Can you work these out from the drawing? Everything is in mm from the part's minimum corner. A direction names the side the tool comes from. Coordinates: 2 decimals unless noted, no trailing zeros. Write each loop counter-clockwise with the first axis right and the second up, starting at its lowest first coordinate (ties: lowest second). Pieces come first, ordered by that corner, then holes. Notation, with made-up numbers: (5.25, -0.75) -> (51.25, -0.75) arc R26 cw to (51.25, 35.25) -> close; hole circle Ø3 at (81, 16.25). An arc over 180 degrees is marked (long way). Use a Markdown table: item, result. Add a question column.
Item 1: Imagine slicing it at C-C, the plane y = 9. Write out the boundary of the cut face in (x, z), and give its area (4 significant figures).
Item 2: Imagine slicing it at A-A, the plane z = 5. Write out the boundary of the cut face in (x, y), and give its area (3 significant figures).
Item 3: If we mould it in two halves opening along X, with no side actions, what happens to the marked faces 1, 2, 3 and 4? For each: pulls with the +X half, pulls with the -X half, needs draft (parallel to the pull), parting line crosses it, or undercut.
Item 4: If I drill on line 1 along X through (y, z) = (5.5, 5.5); line 2 along Z through (x, y) = (5, 3.6); line 3 along Y through (x, z) = (3.75, 2.25), over which ranges is the centre line in solid material (lowest first)? Write a range as from..to.
Item 5: Imagine slicing it at B-B, the plane x = 5. Write out the boundary of the cut face in (y, z), and give its area (3 significant figures).
Item 6: Will these pins go through, and if not, where does the flat tip stop? pin 1 Ø5.5 at (x, z) = (5, 6) entering from +Y; pin 2 Ø6 at (y, z) = (1.5, 8.5) entering from -X; pin 3 Ø1 at (x, y) = (7.5, 2.5) entering from +Z.
Item 7: On a 3-axis mill with a long thin cutter (end or side, diameter ignored), from which of +Z, -Z, +X, -X, +Y, -Y can I reach the whole of each face in a straight line? I mean the marked faces 5, 6 and 7. Say none if no direction works.
Item 8: Imagine slicing it at D-D, the plane y = 1. Write out the boundary of the cut face in (x, z), and give its area (3 significant figures).
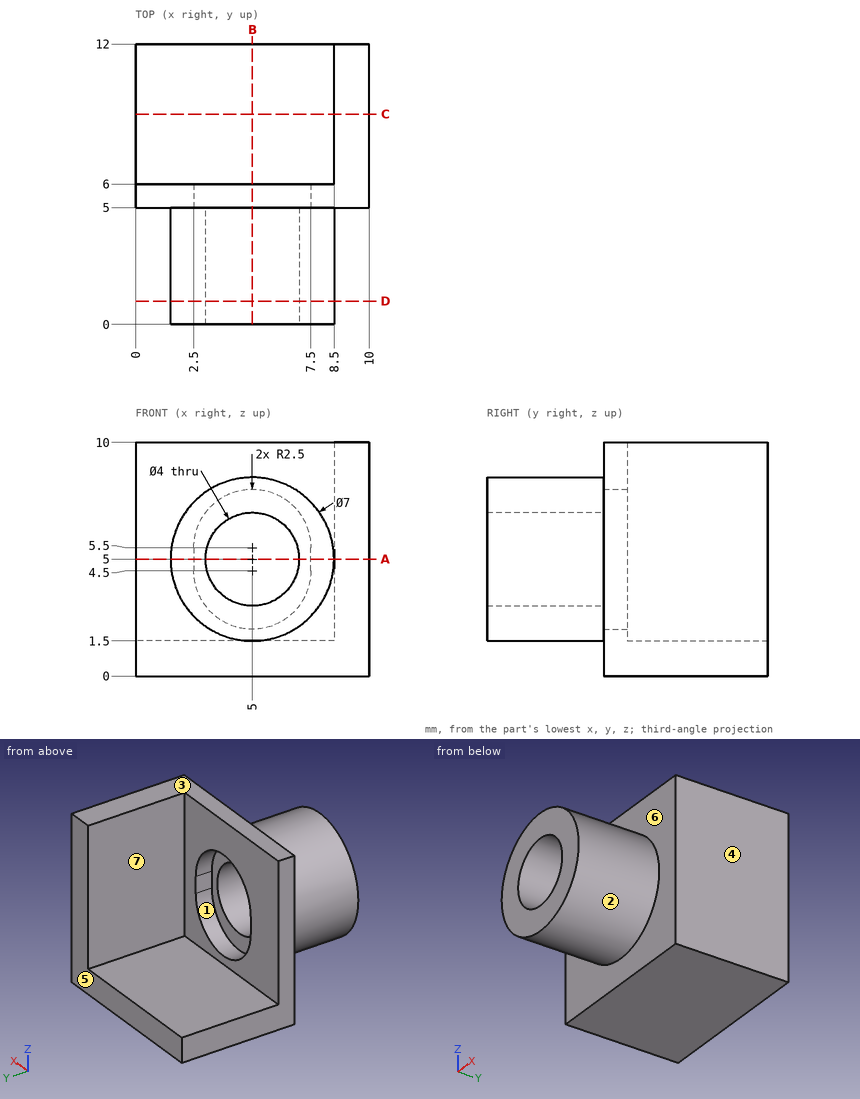
Ans:
| question | item | result |
|---|---|---|
| 1 | outline | (0, 0) -> (10, 0) -> (10, 10) -> (8.5, 10) -> (8.5, 1.5) -> (0, 1.5) -> close |
| 1 | area | 27.75 mm^2 |
| 2 | outline | (0, 5) -> (1.5, 5) -> (1.5, 0) -> (3, 0) -> (3, 5) -> (2.5, 5) -> (2.5, 6) -> (0, 6) -> close; (7, 0) -> (8.5, 0) -> (8.5, 5) -> (10, 5) -> (10, 12) -> (8.5, 12) -> (8.5, 6) -> (7.5, 6) -> (7.5, 5) -> (7, 5) -> close |
| 2 | area | 29.0 mm^2 |
| 3 | face 1 | undercut |
| 3 | face 2 | parting line crosses it |
| 3 | face 3 | needs draft |
| 3 | face 4 | pulls with the +X half |
| 4 | line 1 | x = 0..2.5, 7.5..10 |
| 4 | line 2 | z = 1.5..3, 7..8.5 |
| 4 | line 3 | y = 0..6 |
| 5 | outline | (0, 1.5) -> (5, 1.5) -> (5, 0) -> (12, 0) -> (12, 1.5) -> (6, 1.5) -> (6, 2) -> (5, 2) -> (5, 3) -> (0, 3) -> close; (0, 7) -> (5, 7) -> (5, 8) -> (6, 8) -> (6, 10) -> (5, 10) -> (5, 8.5) -> (0, 8.5) -> close |
| 5 | area | 28.0 mm^2 |
| 6 | pin 1 | stops at y = 6 |
| 6 | pin 2 | stops at x = 1.54 |
| 6 | pin 3 | stops at z = 7.87 |
| 7 | face 5 | +Z, -Z, +X, -X, +Y |
| 7 | face 6 | -Y |
| 7 | face 7 | +Z, -X, +Y |
| 8 | outline | circle Ø7 at (5, 5); hole circle Ø4 at (5, 5) |
| 8 | area | 25.9 mm^2 |
